Verification items for the finished model (mm, model axes). A direction names the side the tool comes from. Give positions to 0.01 mm unless a question says otherwise; leave off trailing zeros. Loops run counter-clockwise (first coordinate to the right, second up) from the corner with the lowest first, then second, coordinate; pieces in that order, holes last. Notation, with made-up numbers: (83, 0.25) - (97, 0.25) arc R19 ccw to (97, 35.25) - close; hole circle Ø1 at (7.5, -21). An arc over 180 degrees is marked (long way). One line per item, written item: value. Start each with the question number.
1. Access from +Z, -Z, +X, -X, +Y, -Y to the whole of each face (thin tool, end or side, straight path). Record for faces 1 (the flat face through (2, 6, 0)), 2 (the cylindrical face through (-1.19, -5.37, 30.82)), 3 (the cylindrical face through (-5.158, -3.955, 34.087)).
2. Sectioned sample at A-A (x = 0). Record the cut outline in (y, z), plus the area to 3 significant figures.
3. Sectioned sample at B-B (z = 11). Record the cut outline in (x, y), plus the area to 3 significant figures.
4. Scan lines: L1, parallel to Y at x = 0, z = 58; L2, parallel to Z at x = 1.75, y = 5; L3, parallel to Z at x = 2, y = -6.5. Record each from-to range of solid material in increasing order. Write a range as [from, to].
5. Gauge pin test, flat ends, axial feed: pin 1 (8 mm diameter, centred on x = -3, z = 43, fed in from +Y); pin 2 (5 mm diameter, centred on x = -3, z = 53, fed in from -Y); pin 3 (8 mm diameter, centred on y = 3.5, z = 43, fed in from +X). Record the tip position at first contact, or that the pin passes through.
6. Mould release check, pull along Y, two halves, no side actions. Record for faces 4 (the flat face through (0, 0, 64)), 5 (the flat face through (0, 0, 62)), 6 (the cylindrical face through (-7.493, 0.33, 2.465)): pulls with the +Y half, pulls with the -Y half, needs draft (parallel to the pull), parting line crosses it, or undercut.
from build123d import *

# Parameters (mm, degrees)
F0_R     = 6.5
F0_R_2   = 5.5
F1_DEPTH = 62
F2_R     = 6.5
F3_DEPTH = 2
F4_R     = 7.5
F4_R_2   = 6.5
F5_DEPTH = 5
F6_R     = 0.5


with BuildPart() as f1:
    # F0 (on Top) → F1 (new body)
    with BuildSketch(Plane.XY):
        Circle(F0_R)
        Circle(F0_R_2, mode=Mode.SUBTRACT)
    extrude(amount=F1_DEPTH)

    # F2 (on face) → F3 (join)
    with BuildSketch(Plane.XY.offset(62)):
        Circle(F2_R)
    extrude(amount=F3_DEPTH)

    # F4 (on Top) → F5 (join)
    with BuildSketch(Plane.XY):
        Circle(F4_R)
        Circle(F4_R_2, mode=Mode.SUBTRACT)
    extrude(amount=F5_DEPTH)

    # F6
    f6_edges = [f1.edges().sort_by_distance(p)[0] for p in [
        (-5.5, 0, 0),
    ]]
    fillet(f6_edges, radius=F6_R)


solid = f1.part
Results are:
1. face 1: -Z, +X, -X, +Y, -Y
1. face 2: -Z
1. face 3: +Z
2. outline: (-7.5, 0) - (-6, 0) arc R0.5 ccw to (-5.5, 0.5) - (-5.5, 62) - (5.5, 62) - (5.5, 0.5) arc R0.5 ccw to (6, 0) - (7.5, 0) - (7.5, 5) - (6.5, 5) - (6.5, 64) - (-6.5, 64) - (-6.5, 5) - (-7.5, 5) - close
2. area: 160 mm^2
3. outline: circle Ø13 at (0, 0); hole circle Ø11 at (0, 0)
3. area: 37.7 mm^2
4. L1: y = [-6.5, -5.5], [5.5, 6.5]
4. L2: z = [62, 64]
4. L3: z = [0, 5]
5. pin 1: stops at y = 6.5
5. pin 2: stops at y = -6.48
5. pin 3: stops at x = 6.5
6. face 4: needs draft
6. face 5: undercut
6. face 6: parting line crosses it
